Can you work these out from the model? Positions are in its coordinate system, mm. Face numbers are marked on the shaded views. A direction names the side the tool comes from. Round coordinates to 2 decimals unless told otherwise and drop trailing zeros. Order: outer loops, then holes, each group sorted by start corner. A loop starts at its lowest first (then second) coordinate and runs counter-clockwise, first axis right, second up. Notation, with made-up numbers: (80.5, 29) - (95.5, 29) arc R18 cw to (95.5, 34) - close; hole circle Ø2 at (9.25, 17). An arc over 180 degrees is marked (long way). Write item = value, one per line.
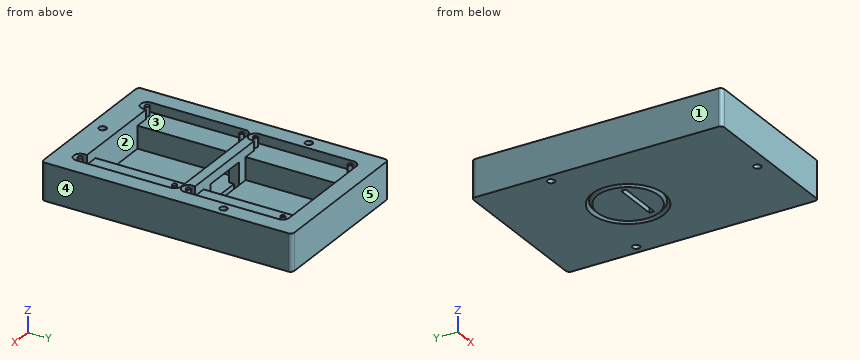
from build123d import *

# Parameters (mm, degrees)
SKETCH_R      = 2
SKETCH_W      = 25
SKETCH_H      = 2.6
PAD_DEPTH     = 3
SKETCH002_R   = 2
PAD001_DEPTH  = 12
SKETCH003_R   = 2
SKETCH003_R_2 = 1.15
PAD002_DEPTH  = 5


with BuildPart() as part:
    # Sketch → Pad (new body)
    with BuildSketch(Plane.XY):
        with BuildLine():
            Line((-42.5, 56.57), (-42.5, -74.85))
            ThreePointArc((-42.5, -74.85), (-41.914214, -76.264214), (-40.5, -76.85))
            Line((-40.5, -76.85), (40.5, -76.85))
            ThreePointArc((40.5, -76.85), (41.914214, -76.264214), (42.5, -74.85))
            Line((42.5, -74.85), (42.5, 56.57))
            ThreePointArc((42.5, 56.57), (41.914214, 57.984214), (40.5, 58.57))
            Line((40.5, 58.57), (-40.5, 58.57))
            ThreePointArc((-40.5, 58.57), (-41.914214, 57.984214), (-42.5, 56.57))
        make_face()
        with Locations((0, -69.85)):
            Circle(SKETCH_R, mode=Mode.SUBTRACT)
        with Locations((37.5, 18.57)):
            Circle(SKETCH_R, mode=Mode.SUBTRACT)
        with Locations((-37.5, 18.57)):
            Circle(SKETCH_R, mode=Mode.SUBTRACT)
        with Locations((0, -5.2)):
            Rectangle(SKETCH_W, SKETCH_H, mode=Mode.SUBTRACT)
    extrude(amount=PAD_DEPTH)

    # Sketch001 → Groove (revolve, cut)
    with BuildSketch(Plane.XZ):
        Polygon((-19.5, 0), (-18, 1.5), (-16.5, 0), align=None)
    revolve(axis=Axis((0, 0, 0), (0, 0, 1)), mode=Mode.SUBTRACT)

    # Sketch002 (on Face5 of Groove) → Pad001 (join)
    with BuildSketch(Plane.XY.offset(3)):
        with BuildLine():
            Line((-42.5, 56.57), (-42.5, -74.85))
            ThreePointArc((-42.5, -74.85), (-41.914214, -76.264214), (-40.5, -76.85))
            Line((-40.5, -76.85), (40.5, -76.85))
            ThreePointArc((40.5, -76.85), (41.914214, -76.264214), (42.5, -74.85))
            Line((42.5, -74.85), (42.5, 56.57))
            ThreePointArc((42.5, 56.57), (41.914214, 57.984214), (40.5, 58.57))
            Line((40.5, 58.57), (-40.5, 58.57))
            ThreePointArc((-40.5, 58.57), (-41.914214, 57.984214), (-42.5, 56.57))
        make_face()
        with Locations((-37.5, 18.57)):
            Circle(SKETCH002_R, mode=Mode.SUBTRACT)
        with Locations((37.5, 18.57)):
            Circle(SKETCH002_R, mode=Mode.SUBTRACT)
        with Locations((0, -69.85)):
            Circle(SKETCH002_R, mode=Mode.SUBTRACT)
        Polygon((-18.5, -62.35), (18.5, -62.35), (18.5, -9.35), (12.5, -9.35), (12.5, -3.93), (18.5, -3.93), (18.5, 49.07), (-18.5, 49.07), (-18.5, -3.93), (-12.5, -3.93), (-12.5, -9.35), (-18.5, -9.35), align=None, mode=Mode.SUBTRACT)
    extrude(amount=PAD001_DEPTH)

    # Sketch003 (on Face17 of Pad001) → Pad002 (join)
    with BuildSketch(Plane.XY.offset(15)):
        with BuildLine():
            Line((-42.5, 56.57), (-42.5, -74.85))
            ThreePointArc((-42.5, -74.85), (-41.914214, -76.264214), (-40.5, -76.85))
            Line((-40.5, -76.85), (40.5, -76.85))
            ThreePointArc((40.5, -76.85), (41.914214, -76.264214), (42.5, -74.85))
            Line((42.5, -74.85), (42.5, 56.57))
            ThreePointArc((42.5, 56.57), (41.914214, 57.984214), (40.5, 58.57))
            Line((40.5, 58.57), (-40.5, 58.57))
            ThreePointArc((-40.5, 58.57), (-41.914214, 57.984214), (-42.5, 56.57))
        make_face()
        with Locations((-37.5, 18.57)):
            Circle(SKETCH003_R, mode=Mode.SUBTRACT)
        with Locations((37.5, 18.57)):
            Circle(SKETCH003_R, mode=Mode.SUBTRACT)
        with Locations((0, -69.85)):
            Circle(SKETCH003_R, mode=Mode.SUBTRACT)
        with BuildLine():
            Line((-33, 45.57), (-33, -5.43))
            ThreePointArc((-33, -5.43), (-29.5, -8.93), (-26, -5.43))
            Line((-26, -5.43), (-26, -3.93))
            Line((-26, -3.93), (26, -3.93))
            Line((26, -3.93), (26, -5.43))
            ThreePointArc((26, -5.43), (29.5, -8.93), (33, -5.43))
            Line((33, -5.43), (33, 45.57))
            ThreePointArc((33, 45.57), (31.974874, 48.044874), (29.5, 49.07))
            Line((29.5, 49.07), (-29.5, 49.07))
            ThreePointArc((-29.5, 49.07), (-31.974874, 48.044874), (-33, 45.57))
        make_face(mode=Mode.SUBTRACT)
        with BuildLine():
            Line((-33, -12.85), (-33, -63.85))
            ThreePointArc((-33, -63.85), (-29.5, -67.35), (-26, -63.85))
            Line((-26, -63.85), (-26, -62.35))
            Line((-26, -62.35), (25.967625, -62.35))
            Line((25.967625, -62.35), (26.000776, -63.923713))
            ThreePointArc((26.000776, -63.923713), (29.536859, -67.349806), (33, -63.85))
            Line((33, -63.85), (33, -12.85))
            ThreePointArc((33, -12.85), (31.974874, -10.375126), (29.5, -9.35))
            Line((29.5, -9.35), (-29.5, -9.35))
            ThreePointArc((-29.5, -9.35), (-31.974874, -10.375126), (-33, -12.85))
        make_face(mode=Mode.SUBTRACT)
        with Locations((-29.5, 45.57)):
            Circle(SKETCH003_R_2)
        with Locations((29.5, 45.57)):
            Circle(SKETCH003_R_2)
        with Locations((-29.5, -5.43)):
            Circle(SKETCH003_R_2)
        with Locations((29.5, -12.85)):
            Circle(SKETCH003_R_2)
        with Locations((29.5, -63.85)):
            Circle(SKETCH003_R_2)
        with Locations((-29.5, -63.85)):
            Circle(SKETCH003_R_2)
        with Locations((-29.5, -12.85)):
            Circle(SKETCH003_R_2)
        with Locations((29.5, -5.43)):
            Circle(SKETCH003_R_2)
    extrude(amount=PAD002_DEPTH)


solid = part.part
(1) If we section it at C-C (y = 0): Write out the boundary of the cut face in (x, z), plus the area to 4 significant figures.
Computed:
outline = (-42.5, 0) - (-19.5, 0) - (-18, 1.5) - (-16.5, 0) - (16.5, 0) - (18, 1.5) - (19.5, 0) - (42.5, 0) - (42.5, 20) - (33, 20) - (33, 15) - (18.5, 15) - (18.5, 3) - (-18.5, 3) - (-18.5, 15) - (-33, 15) - (-33, 20) - (-42.5, 20) - close
area = 921.5 mm^2
(2) If I drill on line 1 (Y direction, x = 0, z = 14.5); line 2 (Y direction, x = -6, z = 19); line 3 (Y direction, x = -1.5, z = 16), over which ranges is the centre line in solid material (lowest first)? Write a range as from..to.
Computed:
line_1 = -76.85..-71.85, -67.85..-62.35, 49.07..58.57
line_2 = -76.85..-62.35, -9.35..-3.93, 49.07..58.57
line_3 = -76.85..-71.17, -68.53..-62.35, -9.35..-3.93, 49.07..58.57
(3) Thinking about a two-plate mould opening in X: for the marked faces 3, 4 and 5, which applies, +X half, -X half, draft (parallel to the pull), parting line (faces both ways), or undercut?
Computed:
face_3 = undercut
face_4 = +X half
face_5 = draft
(4) On a 3-axis mill with a long thin cutter (end or side, diameter ignored), from which of +Z, -Z, +X, -X, +Y, -Y can I reach the whole of each face in a straight line? I mean the marked faces 1 and 2. Say none if no direction works.
Computed:
face_1 = +Z, -Z, -X, +Y, -Y
face_2 = +Z
(5) If we section it at A-A (x = 0): Write out the boundary of the cut face in (y, z).
Computed:
outline = (-76.85, 0) - (-71.85, 0) - (-71.85, 20) - (-76.85, 20) - close; (-67.85, 0) - (-19.5, 0) - (-18, 1.5) - (-16.5, 0) - (-6.5, 0) - (-6.5, 3) - (-62.35, 3) - (-62.35, 20) - (-67.85, 20) - close; (-9.35, 15) - (-3.93, 15) - (-3.93, 20) - (-9.35, 20) - close; (-3.9, 0) - (16.5, 0) - (18, 1.5) - (19.5, 0) - (58.57, 0) - (58.57, 20) - (49.07, 20) - (49.07, 3) - (-3.9, 3) - close
(6) If we section it at D-D (z = 6.25): Write out the boundary of the cut face in (x, y), plus the area to 3 significant figures.
Computed:
outline = (-42.5, -74.85) arc R2 ccw to (-40.5, -76.85) - (40.5, -76.85) arc R2 ccw to (42.5, -74.85) - (42.5, 56.57) arc R2 ccw to (40.5, 58.57) - (-40.5, 58.57) arc R2 ccw to (-42.5, 56.57) - close; hole circle Ø4 at (-37.5, 18.57); hole (-18.5, -62.35) - (18.5, -62.35) - (18.5, -9.35) - (12.5, -9.35) - (12.5, -3.93) - (18.5, -3.93) - (18.5, 49.07) - (-18.5, 49.07) - (-18.5, -3.93) - (-12.5, -3.93) - (-12.5, -9.35) - (-18.5, -9.35) - close; hole circle Ø4 at (0, -69.85); hole circle Ø4 at (37.5, 18.57)
area = 7,410 mm^2
(7) If we section it at B-B (x = -37.5): Write out the boundary of the cut face in (y, z), plus the area to 3 significant figures.
Computed:
outline = (-76.85, 0) - (16.57, 0) - (16.57, 20) - (-76.85, 20) - close; (20.57, 0) - (58.57, 0) - (58.57, 20) - (20.57, 20) - close
area = 2,630 mm^2
(8) Will this pin go through, and if not, where does the flat tip stop? P1, Ø10, axis at x = -16.5, y = -50.5, coming from the +Z side.
Computed:
P1 = 15
